Geometry check sheet. Reference: the model listing, model coordinates, mm. A direction names the side the tool comes from. Give positions to 0.01 mm unless a question says otherwise; leave off trailing zeros. Write each loop counter-clockwise with the first axis right and the second up, starting at its lowest first coordinate (ties: lowest second). Pieces come first, ordered by that corner, then holes. Notation, with made-up numbers: (-3.5, 21.25) - (37.5, 21.25) arc R7 cw to (37.5, 25.25) - close; hole circle Ø4 at (23.5, 11). An arc over 180 degrees is marked (long way). Use a Markdown table: item, result.
```python
from build123d import *

# Parameters (mm, degrees)
SKETCH1_W           = 280
SKETCH1_H           = 100
SKETCH1_R           = 2
SKETCH1_R_2         = 16
BOSS_EXTRUDE1_DEPTH = 10
SKETCH2_R           = 2.75
CUT_EXTRUDE1_DEPTH  = 11
SKETCH3_R           = 4.5
CUT_EXTRUDE2_DEPTH  = 5
CUT_EXTRUDE3_DEPTH  = 11
FILLET1_R           = 10
FILLET2_R           = 5
SKETCH5_R           = 2.75
CUT_EXTRUDE4_DEPTH  = 11
SKETCH6_R           = 4.5
CUT_EXTRUDE5_DEPTH  = 5


with BuildPart() as part:
    # Sketch1 → Boss-Extrude1 (new body)
    with BuildSketch(Plane.XY):
        with Locations((140, 50)):
            Rectangle(SKETCH1_W, SKETCH1_H)
        with Locations((180, 60)):
            Circle(SKETCH1_R, mode=Mode.SUBTRACT)
        with Locations((180, 40)):
            Circle(SKETCH1_R, mode=Mode.SUBTRACT)
        with Locations((100, 60)):
            Circle(SKETCH1_R, mode=Mode.SUBTRACT)
        with Locations((100, 40)):
            Circle(SKETCH1_R, mode=Mode.SUBTRACT)
        with Locations((140, 50)):
            Circle(SKETCH1_R_2, mode=Mode.SUBTRACT)
    extrude(amount=BOSS_EXTRUDE1_DEPTH)

    # Sketch2 → Cut-Extrude1 (cut, through all)
    with BuildSketch(Plane(origin=(0, 0, 0), x_dir=(-1, 0, 0), z_dir=(0, 0, -1))):
        with Locations((-15, 35)):
            Circle(SKETCH2_R)
        with Locations((-15, 65)):
            Circle(SKETCH2_R)
        with Locations((-265, 35)):
            Circle(SKETCH2_R)
        with Locations((-265, 65)):
            Circle(SKETCH2_R)
    extrude(amount=-CUT_EXTRUDE1_DEPTH, mode=Mode.SUBTRACT)

    # Sketch3 → Cut-Extrude2 (cut)
    with BuildSketch(Plane(origin=(0, 0, 0), x_dir=(-1, 0, 0), z_dir=(0, 0, -1))):
        with Locations((-265, 65)):
            Circle(SKETCH3_R)
        with Locations((-265, 35)):
            Circle(SKETCH3_R)
        with Locations((-15, 35)):
            Circle(SKETCH3_R)
        with Locations((-15, 65)):
            Circle(SKETCH3_R)
    extrude(amount=-CUT_EXTRUDE2_DEPTH, mode=Mode.SUBTRACT)

    # Sketch4 → Cut-Extrude3 (cut, through all)
    with BuildSketch(Plane.XY.offset(10)):
        Polygon((10, 25), (30, 25), (30, 75), (10, 75), (10, 90), (130, 90), (130, 75), (85, 75), (85, 25), (130, 25), (130, 10), (10, 10), align=None)
        Polygon((150, 90), (150, 75), (195, 75), (195, 25), (150, 25), (150, 10), (270, 10), (270, 25), (250, 25), (250, 75), (270, 75), (270, 90), align=None)
    extrude(amount=-CUT_EXTRUDE3_DEPTH, mode=Mode.SUBTRACT)

    # Fillet1
    fillet1_edges = [part.edges().sort_by_distance(p)[0] for p in [
        (250, 75, 5),
        (250, 25, 5),
        (195, 25, 5),
        (195, 75, 5),
        (30, 25, 5),
        (30, 75, 5),
        (85, 75, 5),
        (85, 25, 5),
    ]]
    fillet(fillet1_edges, radius=FILLET1_R)

    # Fillet2
    fillet2_edges = [part.edges().sort_by_distance(p)[0] for p in [
        (150, 90, 5),
        (270, 90, 5),
        (270, 75, 5),
        (270, 25, 5),
        (270, 10, 5),
        (150, 10, 5),
        (150, 25, 5),
        (150, 75, 5),
        (10, 10, 5),
        (10, 25, 5),
        (10, 75, 5),
        (10, 90, 5),
        (130, 90, 5),
        (130, 75, 5),
        (130, 25, 5),
        (130, 10, 5),
    ]]
    fillet(fillet2_edges, radius=FILLET2_R)

    # Sketch5 → Cut-Extrude4 (cut, through all)
    with BuildSketch(Plane.XY.offset(10)):
        with Locations((140, 7)):
            Circle(SKETCH5_R)
        with Locations((140, 93)):
            Circle(SKETCH5_R)
    extrude(amount=-CUT_EXTRUDE4_DEPTH, mode=Mode.SUBTRACT)

    # Sketch6 → Cut-Extrude5 (cut)
    with BuildSketch(Plane(origin=(0, 0, 0), x_dir=(-1, 0, 0), z_dir=(0, 0, -1))):
        with Locations((-140, 7)):
            Circle(SKETCH6_R)
        with Locations((-140, 93)):
            Circle(SKETCH6_R)
    extrude(amount=-CUT_EXTRUDE5_DEPTH, mode=Mode.SUBTRACT)


solid = part.part
```
1) Section check B-B on x = 72. Record the boundary of the cut face in (y, z), then the cut area to 3 significant figures.
Working result:
| item | result |
|---|---|
| outline | (0, 0) - (10, 0) - (10, 10) - (0, 10) - close; (90, 0) - (100, 0) - (100, 10) - (90, 10) - close |
| area | 200 mm² |
2) Section check D-D on y = 77.5. Record the boundary of the cut face in (x, z).
Working result:
| item | result |
|---|---|
| outline | (0, 0) - (10.67, 0) - (10.67, 10) - (0, 10) - close; (129.33, 0) - (150.67, 0) - (150.67, 10) - (129.33, 10) - close; (269.33, 0) - (280, 0) - (280, 10) - (269.33, 10) - close |
3) Depth check by flat-ended pin: P1, Ø4.5, axis at x = 16, y = 35, coming from the -Z side; P2, Ø5, axis at x = 265, y = 35, coming from the -Z side. Enter the tip coordinate at first touch or a pass-through.
Working result:
| item | result |
|---|---|
| P1 | stops at z = 5 |
| P2 | passes through |
4) Material ranges on L1, parallel to Y at x = 265, z = 7.8; L2, parallel to Y at x = 162.5, z = 1; L3, parallel to X at y = 15, z = 1, recorded low to high. Write a range as from..to.
Working result:
| item | result |
|---|---|
| L1 | y = 0..10, 25..32.25, 37.75..62.25, 67.75..75, 90..100 |
| L2 | y = 0..10, 25..75, 90..100 |
| L3 | x = 0..10, 130..150, 270..280 |
5) Section check C-C on y = 50. Record the boundary of the cut face in (x, z), then the cut area to 3 significant figures.
Working result:
| item | result |
|---|---|
| outline | (0, 0) - (30, 0) - (30, 10) - (0, 10) - close; (85, 0) - (124, 0) - (124, 10) - (85, 10) - close; (156, 0) - (195, 0) - (195, 10) - (156, 10) - close; (250, 0) - (280, 0) - (280, 10) - (250, 10) - close |
| area | 1,380 mm² |
6) Set-up check for faces 1 (the cylindrical face through (252.85, 71.99, 4.93)), 2 (the cylindrical face through (15.98, 30.61, 2.46)): record each of +Z, -Z, +X, -X, +Y, -Y from which the full face is reachable in a straight line by a thin tool's end or side.
Working result:
| item | result |
|---|---|
| face 1 | +Z, -Z |
| face 2 | -Z |
7) Section check A-A on x = 140. Record the boundary of the cut face in (y, z), then the cut area to 3 significant figures.
Working result:
| item | result |
|---|---|
| outline | (0, 0) - (2.5, 0) - (2.5, 5) - (4.25, 5) - (4.25, 10) - (0, 10) - close; (9.75, 5) - (11.5, 5) - (11.5, 0) - (34, 0) - (34, 10) - (9.75, 10) - close; (66, 0) - (88.5, 0) - (88.5, 5) - (90.25, 5) - (90.25, 10) - (66, 10) - close; (95.75, 5) - (97.5, 5) - (97.5, 0) - (100, 0) - (100, 10) - (95.75, 10) - close |
| area | 535 mm² |
8) Mould release check, pull along Y, two halves, no side actions. Record for faces 3 (the flat face through (138, 73, 10)), 4 (the flat face through (138, 100, 5)), 5 (the cylindrical face through (152, 76, 5)): pulls with the +Y half, pulls with the -Y half, needs draft (parallel to the pull), parting line crosses it, or undercut.
Working result:
| item | result |
|---|---|
| face 3 | needs draft |
| face 4 | pulls with the +Y half |
| face 5 | undercut |
